from build123d import *

# Parameters (mm, degrees)
SKETCH1_R               = 2.4
SKETCH1_R_2             = 2.5
BOSS_EXTRUDE1_DEPTH     = 6
SKETCH2_R               = 1.25
CUT_EXTRUDE1_DEPTH      = 1
CUT_EXTRUDE1_DEPTH_BACK = 11


with BuildPart() as part:
    # Sketch1 → Boss-Extrude1 (new body)
    with BuildSketch(Plane.XY):
        with BuildLine():
            Line((-39.716981132, 22.452830189), (10.283018868, 22.452830189))
            ThreePointArc((10.283018868, 22.452830189), (15.283018868, 17.452830189), (10.283018868, 12.452830189))
            Line((10.283018868, 12.452830189), (-39.716981132, 12.452830189))
            ThreePointArc((-39.716981132, 12.452830189), (-44.716981132, 17.452830189), (-39.716981132, 22.452830189))
        make_face()
        with Locations((10.283018868, 17.452830189)):
            Circle(SKETCH1_R, mode=Mode.SUBTRACT)
        with Locations((-39.716981132, 17.452830189)):
            Circle(SKETCH1_R_2, mode=Mode.SUBTRACT)
    extrude(amount=BOSS_EXTRUDE1_DEPTH)

    # Sketch2 → Cut-Extrude1 (cut, two sides)
    with BuildSketch(Plane(origin=(0, 22.452830189, 0), x_dir=(1, 0, 0), z_dir=(0, 1, 0))) as cut_extrude1_sk:
        with Locations((-39.716981132, -3)):
            Circle(SKETCH2_R)
        with Locations((10.283018868, -3)):
            Circle(SKETCH2_R)
    extrude(amount=CUT_EXTRUDE1_DEPTH, mode=Mode.SUBTRACT)
    extrude(cut_extrude1_sk.sketch, amount=-CUT_EXTRUDE1_DEPTH_BACK, mode=Mode.SUBTRACT)


solid = part.part
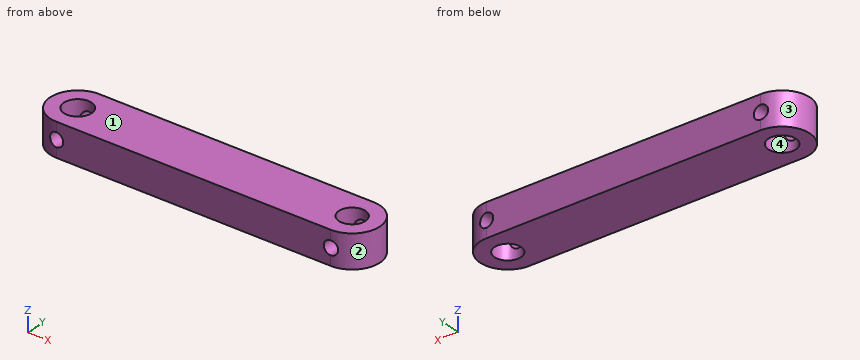
Build history of the part. All positions in model axes, mm. Face numbers are marked on the shaded views. Give positions to 0.01 mm unless a question says otherwise; leave off trailing zeros. Order: outer loops, then holes, each group sorted by start corner. A loop starts at its lowest first (then second) coordinate and runs counter-clockwise, first axis right, second up. Notation, with made-up numbers: M 77,-8 L 115,-8 A23 cw 115,5 Z; hole C 79.5,69 d1. An arc over 180 degrees is marked long. Use one line per item in the form item = value.
Q1. Slice it at B-B, the plane z = 3. Write the cut outline in (x, y), and give its area (3 significant figures).
Conclusion:
outline = M -40.97,12.61 L -40.97,15.29 A2.5 cw -40.97,19.62 L -40.97,22.29 A5 ccw Z; M -38.47,12.45 L 9.03,12.45 L 9.03,15.4 A2.4 cw 9.03,19.5 L 9.03,22.45 L -38.47,22.45 L -38.47,19.62 A2.5 cw -38.47,15.29 Z; M 11.53,12.61 A5 ccw 11.53,22.29 L 11.53,19.5 A2.4 cw 11.53,15.4 Z
area = 514 mm2
Q2. Slice it at A-A, the plane y = 18.5. Write the cut outline in (x, z).
Conclusion:
outline = M -44.61,0 L -41.99,0 L -41.99,6 L -44.61,6 Z; M -37.45,0 L 8.12,0 L 8.12,6 L -37.45,6 Z; M 12.44,0 L 15.17,0 L 15.17,6 L 12.44,6 Z
Q3. Slice it at C-C, the plane y = 14. Write the cut outline in (x, z), and give its area (3 significant figures).
Conclusion:
outline = M -43.33,0 L 13.9,0 L 13.9,6 L -43.33,6 Z; hole C -39.72,3 d2.5; hole C 10.28,3 d2.5
area = 334 mm2
Q4. Wall check: probe 1 along X at (y, z) = (18, 3.75); probe 2 along X at (y, z) = (16.75, 4.5); probe 3 along Y at (x, z) = (-37.5, 4.75). Give the ranges that are in metal, low to high.
Conclusion:
probe_1 = -44.69 to -42.16, -37.28 to 7.95, 12.62 to 15.25
probe_2 = -44.67 to -42.12, -37.32 to 7.99, 12.58 to 15.23
probe_3 = 12.45 to 16.3, 18.61 to 22.45
Q5. Pull direction X, two halves, no side cores. Call the marked faces 1, 2, 3 and 4: released by +X, released by -X, zero draft, split by the parting line, or undercut.
Conclusion:
face_1 = zero draft
face_2 = released by +X
face_3 = released by -X
face_4 = undercut
Q6. Pin check, flat tips, straight feed: P1, Ø1, axis at y = 16, z = 1, coming from the +X side; P2, Ø2, axis at x = 10.28, z = 3, coming from the -Y side; P3, Ø1.5, axis at y = 20.5, z = 1, coming from the +X side. Stop position of each tip, or through.
Conclusion:
P1 = 15.19
P2 = through
P3 = 14.72
